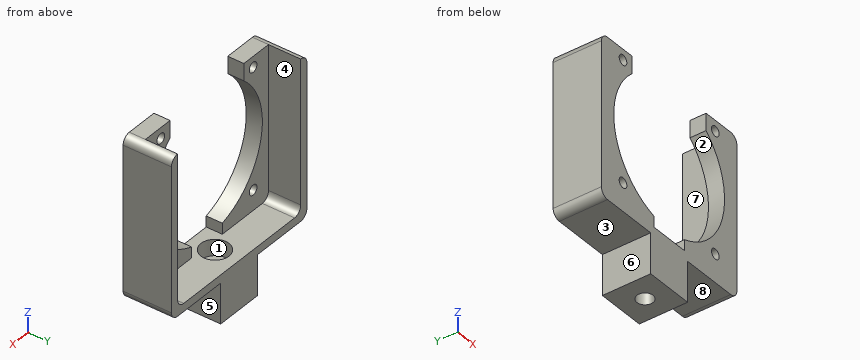
Autodesk Inventor part; units mm, degrees
ref_plane "YZ Plane" through (0, 0, 0) normal (1, 0, 0) x (0, 1, 0)
ref_plane "XZ Plane" through (0, 0, 0) normal (0, 1, 0) x (-1, 0, 0)
ref_plane "XY Plane" through (0, 0, 0) normal (0, 0, 1) x (1, 0, 0)
sketch "Sketch1" plane through (0, 0, 0) normal (0, 1, 0) x (-1, 0, 0)
  line L0 (19, 19) -> (-19, 19) construction
  line L1 (-19, 19) -> (-19, -19) construction
  line L2 (-19, -19) -> (19, -19) construction
  line L3 (19, -19) -> (19, 19) construction
  line L4 (19, 19) -> (-19, -19) construction
  line L5 (-19, 19) -> (19, -19) construction
  circle A0 centre (15, -15) radius 1.25
  circle A1 centre (-15, -15) radius 1.25
  circle A2 centre (-15, 15) radius 1.25
  circle A3 centre (15, 15) radius 1.25
  line L6 (-20, 20) -> (-20, -20)
  line L7 (-20, -20) -> (20, -20)
  line L8 (20, -20) -> (20, 20)
  line L9 (20, 20) -> (-20, -20) construction
  line L10 (-20, 20) -> (20, -20) construction
  line L11 (-22, 22) -> (-22, -22)
  line L12 (-22, -22) -> (22, -22)
  line L13 (22, -22) -> (22, 22)
  line L14 (22, 22) -> (-22, -22) construction
  line L15 (-22, 22) -> (22, -22) construction
  line L16 (12, 13.4164) -> (12, 22)
  line L17 (-12, 13.4164) -> (-12, 22)
  line L18 (20, 20) -> (12, 20)
  line L19 (-12, 20) -> (-20, 20)
  line L20 (22, 22) -> (12, 22)
  line L21 (-12, 22) -> (-22, 22)
  line L22 (5, -17.2916) -> (5, -20)
  line L23 (-5, -20) -> (-5, -17.2916)
  arc A4 (-12, 13.4164) -> (-5, -17.2916) centre (0, 0) ccw
  arc A5 (5, -17.2916) -> (12, 13.4164) centre (0, 0) ccw
  dimension "d0" = 38
  dimension "d1" = 38
  dimension "d2" = 4
  dimension "d3" = 4
  dimension "d4" = 4
  dimension "d5" = 4
  dimension "d6" = 2.5
  dimension "d7" = 2.5
  dimension "d8" = 2.5
  dimension "d9" = 2.5
  dimension "d11" = 40
  dimension "d12" = 40
  dimension "d13" = 44
  dimension "d14" = 44
  dimension "d15" = 10
  dimension "d16" = 10
  dimension "d17" = 17
  dimension "d18" = 17
  dimension "d19" = 18
  dimension "d20" = 18
extrude "Extrusion1" add sketch "Sketch1" along normal blind 4
sketch "Sketch2" plane through (0, 4, 0) normal (0, 1, 0) x (1, 0, 0)
  line L0 (22, 22) -> (-22, 22)
  line L1 (-22, 22) -> (22, 22)
  line L2 (12, -22) -> (22, -22)
  line L3 (22, 22) -> (22, -22)
  line L4 (22, -22) -> (12, -22)
  line L5 (12, -22) -> (12, -20)
  line L6 (12, -20) -> (20, -20)
  line L7 (20, -20) -> (20, 20)
  line L8 (20, 20) -> (-20, 20)
  line L9 (-20, 20) -> (-20, -20)
  line L10 (-22, -22) -> (-12, -22)
  line L11 (-20, 20) -> (20, 20) construction
  line L12 (-20, -20) -> (-12, -20)
  line L13 (-12, -20) -> (-12, -22)
  line L14 (-12, -22) -> (-22, -22)
  line L15 (-22, -22) -> (-22, 22)
  point P0 (0, 0)
  dimension "d23" = 2
  dimension "d24" = 8
  dimension "d25" = 40
  dimension "d26" = 40
  dimension "d27" = 40
  dimension "d28" = 90
extrude "Extrusion2" add sketch "Sketch2" along normal blind 8
sketch "Sketch3" plane through (0, 12, 0) normal (0, 1, 0) x (1, 0, 0)
  line L0 (-24.6321, -17.6536) -> (24.6321, -17.6536)
  line L1 (24.6321, -17.6536) -> (24.6321, -22.4819)
  line L2 (24.6321, -22.4819) -> (-24.6321, -22.4819)
  line L3 (-24.6321, -22.4819) -> (-24.6321, -17.6536)
  line L4 (-24.6321, -17.6536) -> (24.6321, -22.4819) construction
  line L5 (24.6321, -17.6536) -> (-24.6321, -22.4819) construction
  point P0 (0, 0)
  point P1 (0, -20.0678)
extrude "Extrusion3" cut sketch "Sketch3" against normal through all
fillet "Fillet2" radius 2 6 edges at (20, 8, -20) (-20, 8, -20) (-22, 6, 17.6536) (22, 6, 17.6536) (22, 6, -22) (-22, 6, -22)
sketch "Sketch4" plane through (20, 0, -22) normal (0, 0, -1) x (-1, 0, 0)
  line L0 (0, 0) -> (40, 0)
  line L1 (26, 0) -> (14, 0)
  line L2 (14, 0) -> (14, 12)
  line L3 (14, 12) -> (26, 12)
  line L4 (26, 12) -> (26, 0)
  point P0 (20, 0)
  point P1 (20, 0)
  dimension "d35" = 12
  dimension "d36" = 12
  dimension "d37" = 6
extrude "Extrusion4" add sketch "Sketch4" along normal blind 10
sketch "Sketch5" plane through (-5, 0, -20) normal (0, 0, 1) x (1, 0, 0)
  circle A0 centre (5, 6) radius 3.5
  line L0 (-13, 12) -> (23, 12)
  line L1 (27, 0) -> (27, 12)
  point P0 (5, 0)
  dimension "d40" = 7
  dimension "d41" = 6
  dimension "d42" = 22
extrude "Extrusion5" cut sketch "Sketch5" against normal blind 4
sketch "Sketch6" plane through (0, 6, -24) normal (0, 0, 1) x (1, 0, 0)
  circle A0 centre (0, 0) radius 2
  line L0 (-18, 6) -> (18, 6)
  line L1 (22, -6) -> (22, 6)
  point P0 (0, -6)
  dimension "d45" = 4
  dimension "d46" = 6
  dimension "d47" = 22
extrude "Extrusion6" cut sketch "Sketch6" against normal through all
properties part number "CameraMount1"
Work out the finished part from the listing and answer in its coordinate system (mm). Face numbers are marked on the shaded views. A direction names the side the tool comes from. Coordinates: 2 decimals unless noted, no trailing zeros. Order: outer loops, then holes, each group sorted by start corner. A loop starts at its lowest first (then second) coordinate and runs counter-clockwise, first axis right, second up. Notation, with made-up numbers: (84, -36.75) - (97, -36.75) arc R12 cw to (97, -26.75) - close; hole circle Ø5 at (36.25, 65). An arc over 180 degrees is marked (long way). Put each result on its own line as item: value. Start each with the question number.
1) Find section B-B (x = 0). Give the vertices of the cut face in (y, z).
2) Find section A-A (z = 15). Give the vertices of the cut face in (x, y).
3) Find section C-C (y = 6). Give the vertices of the cut face in (x, z), plus the area to 3 significant figures.
4) Find the intervals of material crossed by line 1 (X direction, y = 7, z = -2.5); line 2 (Y direction, x = 0, z = -22.95); line 3 (Z direction, x = -15, y = 2.8), in increasing order. Write a range as from..to.
5) Flat-ended cylindrical pins translate along their axes: pin 1 (3.5 mm diameter, centred on x = -11.5, y = 6.5, fed in from -Z); pin 2 (2 mm diameter, centred on x = 15, z = -15, fed in from +Y); pin 3 (5.5 mm diameter, centred on x = 1, y = 7.5, fed in from +Z); pin 4 (1.5 mm diameter, centred on x = -17.5, z = -14.5, fed in from +Y). Find the tip coordinate at first contact, or state that the pin passes through.
6) For a pull along X with two mould halves and no side action, classify the marked faces 5, 6, 7 and 8 as released by +X, released by -X, zero draft, split by the parting line, or undercut.
7) Find section D-D (z = -27). Give the vertices of the cut face in (x, y).
8) For the marked faces 1, 2, 3 and 4, determine the directions among +Z, -Z, +X, -X, +Y, -Y from which every point of the face is accessible in a straight line to the end or side of a thin tool.
Results list:
1. outline: (0, -32) - (4, -32) - (4, -24) - (2.5, -24) - (2.5, -20) - (0, -20) - close; (8, -32) - (12, -32) - (12, -20) - (9.5, -20) - (9.5, -24) - (8, -24) - close
2. outline: (-22, 0) - (-16.25, 0) - (-16.25, 4) - (-20, 4) - (-20, 12) - (-22, 12) - close; (-13.75, 0) - (-12, 0) - (-12, 4) - (-13.75, 4) - close; (12, 0) - (13.75, 0) - (13.75, 4) - (12, 4) - close; (16.25, 0) - (22, 0) - (22, 12) - (20, 12) - (20, 4) - (16.25, 4) - close
3. outline: (-22, -20) arc R2 ccw to (-20, -22) - (-6, -22) - (-6, -32) - (-2, -32) - (-2, -24) - (-3.5, -24) - (-3.5, -20) - (-18, -20) arc R2 cw to (-20, -18) - (-20, 17.65) arc R2 ccw to (-22, 15.65) - close; (2, -32) - (6, -32) - (6, -22) - (20, -22) arc R2 ccw to (22, -20) - (22, 15.65) arc R2 ccw to (20, 17.65) - (20, -18) arc R2 cw to (18, -20) - (3.5, -20) - (3.5, -24) - (2, -24) - close
3. area: 297 mm^2
4. line 1: x = -22..-20, 20..22
4. line 2: y = 0..2.5, 9.5..12
4. line 3: z = -22..-16.25, -13.75..-9.95, 9.95..13.75, 16.25..17.65
5. pin 1: stops at z = -22
5. pin 2: passes through
5. pin 3: stops at z = -20
5. pin 4: stops at y = 4
6. face 5: released by +X
6. face 6: released by -X
6. face 7: undercut
6. face 8: zero draft
7. outline: (-6, 0) - (6, 0) - (6, 12) - (-6, 12) - close; hole circle Ø4 at (0, 6)
8. face 1: +Z
8. face 2: +Y, -Y
8. face 3: -Z, -X, +Y, -Y
8. face 4: +Z, +Y
